from build123d import *

# Parameters (mm, degrees)
CROQUIS1_R              = 4
CROQUIS1_R_2            = 2.5
CROQUIS1_R_3            = 3.15
SALIENTE_EXTRUIR1_DEPTH = 3


with BuildPart() as part:
    # Croquis1 → Saliente-Extruir1 (new body)
    with BuildSketch(Plane(origin=(0, 0, 0), x_dir=(1, 0, 0), z_dir=(0, 1, 0))):
        with BuildLine():
            Line((25, -37.15), (-25, -37.15))
            Line((-25, -37.15), (-25, 12.85))
            ThreePointArc((-25, 12.85), (-22.071067812, 19.921067812), (-15, 22.85))
            Line((-15, 22.85), (15, 22.85))
            ThreePointArc((15, 22.85), (22.071067812, 19.921067812), (25, 12.85))
            Line((25, 12.85), (25, -37.15))
        make_face()
        with Locations(Location((0, 0, 0), (0, 0, 270))):
            Circle(CROQUIS1_R, mode=Mode.SUBTRACT)
        with Locations(Location((18.25, 0, 0), (0, 0, 270))):
            Circle(CROQUIS1_R_2, mode=Mode.SUBTRACT)
        with Locations(Location((-18.25, 0, 0), (0, 0, 90))):
            Circle(CROQUIS1_R_2, mode=Mode.SUBTRACT)
        with Locations(Location((-10, -24.65, 0), (0, 0, 270))):
            Circle(CROQUIS1_R_3, mode=Mode.SUBTRACT)
        with Locations(Location((10, -24.65, 0), (0, 0, 90))):
            Circle(CROQUIS1_R_3, mode=Mode.SUBTRACT)
    extrude(amount=SALIENTE_EXTRUIR1_DEPTH)


solid = part.part
Work out the finished part from the listing and answer in its coordinate system (mm). Round coordinates to 2 decimals unless told otherwise and drop trailing zeros. Loops run counter-clockwise (first coordinate to the right, second up) from the corner with the lowest first, then second, coordinate; pieces in that order, holes last. Notation, with made-up numbers: M -17.75,22.5 L -11.75,22.5 A34 cw -11.75,55.5 Z; hole C 15,61.25 d4. An arc over 180 degrees is marked long. One line per question, with ' | ' between items. Start each with the question number.
(1) A cutting plane is placed at A-A on x = 0. Write down the section's boundary in (y, z).
(2) Find the intervals of material crossed by line 1 (X direction, y = 1.8, z = 24.65); line 2 (X direction, y = 2.65, z = 0); line 3 (Z direction, x = 7.5, y = 0.3), in increasing order.
(3) For a pull along Z with two mould halves and no side action, classify faces 1 (the face through (-7.9, 1.5, 22.3)), 2 (the face through (25, 1, 12)), 3 (the face through (21.99, 1.48, -20)) as released by +Z, released by -Z, zero draft, split by the parting line, or undercut.
(4) A cutting plane is placed at D-D on z = 24.65. Write down the section's boundary in (x, y), plus the area to 3 significant figures.
(5) A flat-ended cylindrical pin translates along its axis: pin 1 Ø9 at (x, z) = (0, 0) entering from +Y. Find the tip coordinate at first contact, or state that the pin passes through.
(6) A cutting plane is placed at B-B on y = 1.25. Write down the section's boundary in (x, z).
(7) A cutting plane is placed at C-C on z = 0. Write down the section's boundary in (x, y).
Geometry check:
1) outline: M 0,-22.85 L 3,-22.85 L 3,-4 L 0,-4 Z; M 0,4 L 3,4 L 3,37.15 L 0,37.15 Z
2) line 1: x = -25 to -13.15, -6.85 to 6.85, 13.15 to 25 | line 2: x = -25 to -20.75, -15.75 to -4, 4 to 15.75, 20.75 to 25 | line 3: z = -22.85 to 22.73, 26.57 to 37.15
3) face 1: undercut | face 2: zero draft | face 3: released by -Z
4) outline: M -25,0 L -13.15,0 L -13.15,3 L -25,3 Z; M -6.85,0 L 6.85,0 L 6.85,3 L -6.85,3 Z; M 13.15,0 L 25,0 L 25,3 L 13.15,3 Z | area: 112 mm²
5) pin 1: stops at y = 3
6) outline: M -25,-12.85 A10 ccw -15,-22.85 L 15,-22.85 A10 ccw 25,-12.85 L 25,37.15 L -25,37.15 Z; hole C -18.25,0 d5; hole C -10,24.65 d6.3; hole C 0,0 d8; hole C 10,24.65 d6.3; hole C 18.25,0 d5
7) outline: M -25,0 L -20.75,0 L -20.75,3 L -25,3 Z; M -15.75,0 L -4,0 L -4,3 L -15.75,3 Z; M 4,0 L 15.75,0 L 15.75,3 L 4,3 Z; M 20.75,0 L 25,0 L 25,3 L 20.75,3 Z
